Autodesk Inventor part; units mm, degrees
ref_plane "YZ Plane" through (0, 0, 0) normal (1, 0, 0) x (0, 1, 0)
ref_plane "XZ Plane" through (0, 0, 0) normal (0, 1, 0) x (-1, 0, 0)
ref_plane "XY Plane" through (0, 0, 0) normal (0, 0, 1) x (1, 0, 0)
sketch "Sketch1" plane through (0, 0, 0) normal (0, 1, 0) x (-1, 0, 0)
  circle A0 centre (0, 0) radius 12.7
  circle A1 centre (0, 0) radius 20
  dimension "d0" = 25.4
  dimension "d1" = 40
extrude "Extrusion1" add sketch "Sketch1" along normal mid plane 30
fillet "Fillet2" radius 5 2 edges at (20, 15, 0) (20, -15, 0)
sketch "Sketch6" plane through (0, 0, 0) normal (0, 0, 1) x (1, 0, 0)
  circle A0 centre (0, 0) radius 4
  dimension "d33" = 8
extrude "Extrusion6" add sketch "Sketch6" along normal blind 65.4
sketch "Sketch7" plane through (0, 0, 0) normal (0, 1, 0) x (-1, 0, 0)
  circle A0 centre (0, 0) radius 12.7
extrude "Extrusion7" cut sketch "Sketch7" along normal through all both and the other way through all
fillet "Fillet3" radius 1 1 edges at (-4, 0, 65.4)
properties part number "suporte-barra" material "Aluminium AW-7020"
Model file for the job. Use its own axes, mm. A direction names the side the tool comes from. Give positions to 0.01 mm unless a question says otherwise; leave off trailing zeros. Loops run counter-clockwise (first coordinate to the right, second up) from the corner with the lowest first, then second, coordinate; pieces in that order, holes last. Notation, with made-up numbers: (82.5, 12) -> (92.5, 12) arc R12 ccw to (92.5, 32) -> close; hole circle Ø11 at (36, 22.5). An arc over 180 degrees is marked (long way). Use a Markdown table: item, result. Add a question column.
(1) Mould opens along Z. For faces 1 (the cylindrical face through (2.75, 0.21, -12.4)), 2 (the flat face through (0, 0, 65.4)), 3 (the flat face through (11, 15, 7)) say: +Z half, -Z half, draft (parallel to the pull), parting line (faces both ways), or undercut.
(2) Slice it at B-B on x = 0. List the corners of the cut face in (y, z), and give its area (3 significant figures).
(3) Tool access for faces 4 (the flat face through (11, -15, 7)), 5 (the cylindrical face through (-0.867, 3.905, 41.684)): list every direction of +Z, -Z, +X, -X, +Y, -Y with a clear straight run to the whole face (end or side of a thin tool).
(4) Slice it at C-C on y = 0. List the corners of the cut face in (x, z), and give its area (3 significant figures).
(5) Slice it at D-D on z = 44.5. List the corners of the cut face in (x, y), and give its area (3 significant figures).
(6) Slice it at A-A on z = 0. List the corners of the cut face in (x, y).
(7) Wall check: line 1 along Z through (x, y) = (0, 1); line 2 along Z through (x, y) = (0, -4.75); line 3 along X through (y, z) = (-10, -8). Give the ranges that are in metal, low to high.
(8) Drop flat-ended pins along their axis: pin 1 Ø10 at (y, z) = (-3.5, 40.5) entering from -X; pin 2 Ø6 at (y, z) = (2, 3.5) entering from -X; pin 3 Ø2 at (y, z) = (-10, -6.5) entering from -X; pin 4 Ø6 at (y, z) = (-2, 2) entering from +X. Give the stop position or say it passes through.
Filled sheet:
| question | item | result |
|---|---|---|
| 1 | face 1 | undercut |
| 1 | face 2 | +Z half |
| 1 | face 3 | draft |
| 2 | outline | (-15, -15) arc R5 ccw to (-10, -20) -> (10, -20) arc R5 ccw to (15, -15) -> (15, -12.7) -> (-15, -12.7) -> close; (-15, 12.7) -> (15, 12.7) -> (15, 15) arc R5 ccw to (10, 20) -> (4, 20) -> (4, 64.4) arc R1 ccw to (3, 65.4) -> (-3, 65.4) arc R1 ccw to (-4, 64.4) -> (-4, 20) -> (-10, 20) arc R5 ccw to (-15, 15) -> close |
| 2 | area | 779 mm2 |
| 3 | face 4 | +Z, -Z, +X, -X, -Y |
| 3 | face 5 | +Z |
| 4 | outline | (-4, 19.6) arc R20 ccw (long way) to (4, 19.6) -> (4, 64.4) arc R1 ccw to (3, 65.4) -> (-3, 65.4) arc R1 ccw to (-4, 64.4) -> close; hole circle Ø25.4 at (0, 0) |
| 4 | area | 1,110 mm2 |
| 5 | outline | circle Ø8 at (0, 0) |
| 5 | area | 50.3 mm2 |
| 6 | outline | (-20, -10) arc R5 ccw to (-15, -15) -> (-12.7, -15) -> (-12.7, 15) -> (-15, 15) arc R5 ccw to (-20, 10) -> close; (12.7, -15) -> (15, -15) arc R5 ccw to (20, -10) -> (20, 10) arc R5 ccw to (15, 15) -> (12.7, 15) -> close |
| 7 | line 1 | -20 to -12.7, 12.7 to 65.4 |
| 7 | line 2 | -20 to -12.7, 12.7 to 20 |
| 7 | line 3 | -18.33 to -9.86, 9.86 to 18.33 |
| 8 | pin 1 | x = -4 |
| 8 | pin 2 | x = -19.99 |
| 8 | pin 3 | x = -19.23 |
| 8 | pin 4 | x = 20 |
